```python
from build123d import *

# Parameters (mm, degrees)
F1_DEPTH = 6


with BuildPart() as f1:
    # F0 (on Top) → F1 (new body)
    with BuildSketch(Plane.XY):
        with BuildLine():
            ThreePointArc((-0.524037, -3.965525), (2.636651, -3.008002), (4, 0))
            ThreePointArc((4, 0), (-2.636651, 3.008002), (-0.524037, -3.965525))
        make_face()
        with BuildLine():
            ThreePointArc((-50, -110), (-32.075898, -106.82234), (-13.928128, -105.397782))
            ThreePointArc((-13.928128, -105.397782), (4.272256, -105.739751), (22.353704, -107.845026))
            Line((22.353704, -107.845026), (14.980582, 0.76299))
            ThreePointArc((14.980582, 0.76299), (2.035325, 14.861274), (-14.223815, 4.762676))
            Line((-14.223815, 4.762676), (-50, -110))
        make_face()
        with BuildLine():
            ThreePointArc((-12.487026, -94.492589), (-24.532233, -78.779123), (-8.818768, -66.733917))
            ThreePointArc((-8.818768, -66.733917), (-0.124891, -71.384976), (3.347103, -80.613253))
            ThreePointArc((3.347103, -80.613253), (-1.42462, -91.141259), (-12.487026, -94.492589))
        make_face(mode=Mode.SUBTRACT)
        with BuildLine():
            ThreePointArc((-7.639684, -57.811486), (-16.243403, -46.587583), (-5.0195, -37.983864))
            ThreePointArc((-5.0195, -37.983864), (1.190412, -41.306049), (3.670408, -47.897675))
            ThreePointArc((3.670408, -47.897675), (0.262034, -55.417679), (-7.639684, -57.811486))
        make_face(mode=Mode.SUBTRACT)
        with BuildLine():
            ThreePointArc((-3.971426, -30.052814), (-10.424215, -21.634886), (-2.006287, -15.182097))
            ThreePointArc((-2.006287, -15.182097), (2.651147, -17.673736), (4.511144, -22.617456))
            ThreePointArc((4.511144, -22.617456), (1.954863, -28.257459), (-3.971426, -30.052814))
        make_face(mode=Mode.SUBTRACT)
        with BuildLine():
            ThreePointArc((-0.524037, -3.965525), (-2.636651, 3.008002), (4, 0))
            ThreePointArc((4, 0), (2.636651, -3.008002), (-0.524037, -3.965525))
        make_face(mode=Mode.SUBTRACT)
    extrude(amount=F1_DEPTH)


solid = f1.part
```
The listing builds one solid part. Answer for the finished solid, in the listing's coordinates (mm). Give positions to 0.01 mm unless a question says otherwise; leave off trailing zeros. Order: outer loops, then holes, each group sorted by start corner. A loop starts at its lowest first (then second) coordinate and runs counter-clockwise, first axis right, second up. Notation, with made-up numbers: (26, 55.25) - (47, 55.25) arc R29 ccw to (47, 75.25) - close; hole circle Ø7 at (0, 89). An arc over 180 degrees is marked (long way). Use one line per item in the form item = value. Start each with the question number.
(1) Consider line 1 (Y direction, x = 0, z = 4.55); line 2 (Y direction, x = -2, z = 4.3); line 3 (X direction, y = -47.5, z = 2.55). Determine where each line is inside the solid, lowest interval first. Write a range as from..to.
(2) A cutting plane is placed at C-C, the plane x = -19. Write down the section's boundary in (y, z), then the cut area to 3 significant figures.
(3) A cutting plane is placed at B-B, the plane y = -72. Write down the section's boundary in (x, z).
(4) A cutting plane is placed at A-A, the plane z = 2.7. Write down the section's boundary in (x, y), then the cut area to 3 significant figures.
(5) Flat-ended cylindrical pins translate along their axes: pin 1 Ø2 at (y, z) = (-89.5, 1.5) entering from +X; pin 2 Ø3 at (x, z) = (-22, 3) entering from -Y; pin 3 Ø6.5 at (x, y) = (0, 0) entering from +Z. Find the tip coordinate at first contact, or state that the pin passes through.
(6) A cutting plane is placed at D-D, the plane y = 7. Write down the section's boundary in (x, z), then the cut area to 3 significant figures.
Ans:
q1.line_1 = -105.5..-89.7, -71.53..-55.64, -40.16..-29.5, -15.74..-4, 4..15
q1.line_2 = -105.42..-91.62, -69.61..-56.91, -38.88..-30.05, -15.18..-3.46, 3.46..14.87
q1.line_3 = -30.52..-16.32, 3.66..18.26
q2.outline = (-105.62, 0) - (-91.85, 0) - (-91.85, 6) - (-105.62, 6) - close; (-69.37, 0) - (-10.56, 0) - (-10.56, 6) - (-69.37, 6) - close
q2.area = 435 mm^2
q3.outline = (-38.15, 0) - (-21.69, 0) - (-21.69, 6) - (-38.15, 6) - close; (0.38, 0) - (19.92, 0) - (19.92, 6) - (0.38, 6) - close
q4.outline = (-50, -110) arc R187.5 cw to (-13.93, -105.4) arc R187.5 cw to (22.35, -107.85) - (14.98, 0.76) arc R15 ccw to (-14.22, 4.76) - close; hole circle Ø20 at (-6.33, -47.9); hole circle Ø15 at (-2.99, -22.62); hole (-8.82, -66.73) arc R14 ccw (long way) to (3.35, -80.61) arc R14 ccw to start; hole circle Ø8 at (0, 0)
q4.area = 4,630 mm^2
q5.pin_1 = 21.18
q5.pin_2 = -105.93
q5.pin_3 = through
q6.outline = (-13.27, 0) - (13.27, 0) - (13.27, 6) - (-13.27, 6) - close
q6.area = 159 mm^2
